For this review, use the dimensioned drawing (mm, ordinates from the lowest corner) and the shaded views. A direction names the side the tool comes from. Round coordinates to 2 decimals unless told otherwise and drop trailing zeros. Write each loop counter-clockwise with the first axis right and the second up, starting at its lowest first coordinate (ties: lowest second). Pieces come first, ordered by that corner, then holes. Notation, with made-up numbers: M 53,-7 L 112,-7 A22 ccw 112,1 Z; hole C -20.75,-15.75 d3. An arc over 180 degrees is marked long. One line per question, with ' | ' between items. Start each with the question number.
Item 1: Add section B-B, the plane y = 65. State the section outline as (x, z) points.
Item 2: Add section D-D, the plane x = 136.5. State the section outline as (y, z) points, and give its area (3 significant figures).
Item 3: Insertion check: pin 1 Ø12 at (x, y) = (152, 88) entering from +Z; pin 2 Ø1.5 at (x, y) = (173, 79) entering from -Z; pin 3 Ø6 at (y, z) = (107, 89.5) entering from -X. Each pin has a flat end and moves straight along its axis. Give the tip position at first contact, or say it passes through.
Item 4: For L1, parallel to Y at x = 230, z = 81; L2, parallel to Z at x = 254, y = 21; L3, parallel to X at y = 65, z = 63.5, list the stretches that pass through material, from the lowest coordinate up.
Item 5: Machinability: for the marked faces 4, 5, 6, 7 and 8, which of the approach directions +Z, -Z, +X, -X, +Y, -Y give a long, thin tool a straight path to every point of the face, cutting with its end or side? Answer none if there is none.
Item 6: Add section C-C, the plane z = 65. State the section outline as (x, y) points, and give its area (3 significant figures).
Item 7: Draft analysis for pull direction X (two halves, no side actions). For the marked faces 1, 2 and 3, state which applies: released by +X, released by -X, zero draft, split by the parting line, or undercut.
Item 8: Add section A-A, the plane x = 230. State the section outline as (y, z) points, and give its area (3 significant figures).
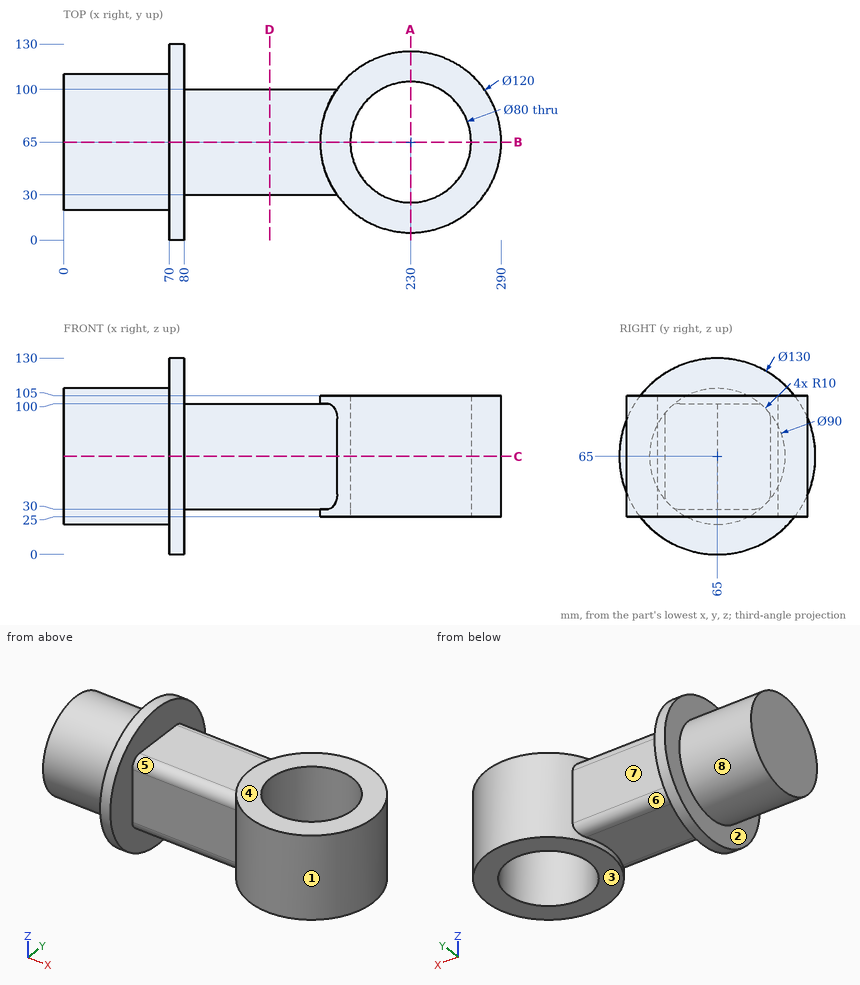
Computed values:
1) outline: M 0,20 L 70,20 L 70,0 L 80,0 L 80,30 L 170,30 L 170,25 L 190,25 L 190,105 L 170,105 L 170,100 L 80,100 L 80,130 L 70,130 L 70,110 L 0,110 Z; M 270,25 L 290,25 L 290,105 L 270,105 Z
2) outline: M 30,40 A10 ccw 40,30 L 90,30 A10 ccw 100,40 L 100,90 A10 ccw 90,100 L 40,100 A10 ccw 30,90 Z | area: 4,810 mm^2
3) pin 1: stops at z = 100 | pin 2: stops at z = 25 | pin 3: stops at x = 70
4) L1: y = 5 to 25, 105 to 125 | L2: z = 25 to 105 | L3: x = 0 to 190, 270 to 290
5) face 4: +Z, +X, +Y, -Y | face 5: +Z, -Y | face 6: -Z, +Y | face 7: +Z, -Z, +Y | face 8: -X
6) outline: M 0,20 L 70,20 L 70,0 L 80,0 L 80,30 L 181.27,30 A60 ccw long 181.27,100 L 80,100 L 80,130 L 70,130 L 70,110 L 0,110 Z; hole C 230,65 d80 | area: 20,400 mm^2
7) face 1: undercut | face 2: released by -X | face 3: zero draft
8) outline: M 5,25 L 25,25 L 25,105 L 5,105 Z; M 105,25 L 125,25 L 125,105 L 105,105 Z | area: 3,200 mm^2
